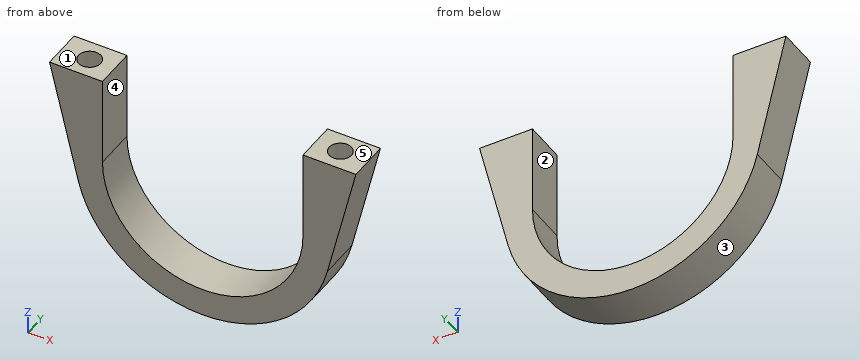
```python
from build123d import *

# Parameters (mm, degrees)
BOSS_EXTRUDE1_DEPTH = 7.5
SKETCH2_R           = 2
CUT_EXTRUDE1_DEPTH  = 4


with BuildPart() as part:
    # Sketch1 → Boss-Extrude1 (new body)
    with BuildSketch(Plane(origin=(0, 0, 0), x_dir=(1, 0, 0), z_dir=(0, 1, 0))):
        with BuildLine():
            Line((-22.363274725, 5.374378434), (-27.5, -16))
            Line((-27.5, -16), (-18, -16))
            Line((-18, -16), (-18, 0))
            ThreePointArc((-18, 0), (0, 18), (18, 0))
            Line((18, 0), (18, -16))
            Line((18, -16), (27.5, -16))
            Line((27.5, -16), (22.363274725, 5.374378434))
            ThreePointArc((22.363274725, 5.374378434), (0, 23), (-22.363274725, 5.374378434))
        make_face()
    extrude(amount=BOSS_EXTRUDE1_DEPTH)

    # Sketch2 → Cut-Extrude1 (cut)
    with BuildSketch(Plane.XY.offset(16)):
        with Locations((-22.5, 3.75)):
            Circle(SKETCH2_R)
        with Locations((22.5, 3.75)):
            Circle(SKETCH2_R)
    extrude(amount=-CUT_EXTRUDE1_DEPTH, mode=Mode.SUBTRACT)


solid = part.part
```
The listing builds one solid part. Answer for the finished solid, in the listing's coordinates (mm). Face numbers are marked on the shaded views. A direction names the side the tool comes from. Coordinates: 2 decimals unless noted, no trailing zeros. Write each loop counter-clockwise with the first axis right and the second up, starting at its lowest first coordinate (ties: lowest second). Pieces come first, ordered by that corner, then holes. Notation, with made-up numbers: (31.5, 77.25) - (78.5, 77.25) arc R22 cw to (78.5, 105.25) - close; hole circle Ø8 at (55, -22.75). An arc over 180 degrees is marked (long way). Return JSON: item names as keys, results as strings. Group by question number.
Q1. The part is cut by section C-C on x = 0. Write down the section's boundary in (y, z).
Q2. Find the intervals of material crossed by line 1 along Y through (x, z) = (22.5, 14.05); line 2 along X through (y, z) = (7, -2.5); line 3 along X through (y, z) = (3.75, -11), in increasing order. Write a range as [from, to].
Q3. Which of the six approach directions +Z, -Z, +X, -X, +Y, -Y give full straight-line access (tool end or side, diameter ignored) to the marked faces 1 and 2?
Q4. The part is cut by section B-B on z = 8.5. Write down the section's boundary in (x, y), and give its area (3 significant figures).
Q5. Flat-ended cylindrical pins translate along their axes: pin 1 Ø4 at (x, y) = (-20.5, 1.5) entering from -Z; pin 2 Ø1.5 at (x, y) = (-6, 4.5) entering from +Z; pin 3 Ø4 at (y, z) = (2.5, 5.5) entering from -X. Find the tip coordinate at first contact, or state that the pin passes through.
Q6. For a pull along X with two mould halves and no side action, classify the marked faces 3, 4 and 5 as +X half, -X half, draft (parallel to the pull), parting line (faces both ways), or undercut.
Q7. The part is cut by section A-A on y = 3.75. Write down the section's boundary in (x, z).
Q8. The part is cut by section D-D on y = 1. Write down the section's boundary in (x, z).
Evaluation:
{
 "1": {"outline": "(0, -23) - (7.5, -23) - (7.5, -18) - (0, -18) - close"},
 "2": {"line 1": "y = [0, 1.75], [5.75, 7.5]", "line 2": "x = [-23.05, -17.83], [17.83, 23.05]", "line 3": "x = [-20.2, -14.25], [14.25, 20.2]"},
 "3": {"face 1": "+Z, +X, -X, +Y, -Y", "face 2": "+Z, +Y, -Y"},
 "4": {"outline": "(-25.7, 0) - (-18, 0) - (-18, 7.5) - (-25.7, 7.5) - close; (18, 0) - (25.7, 0) - (25.7, 7.5) - (18, 7.5) - close", "area": "115 mm2"},
 "5": {"pin 1": "stops at z = -13.67", "pin 2": "stops at z = -16.69", "pin 3": "stops at x = -25.46"},
 "6": {"face 3": "parting line", "face 4": "undercut", "face 5": "draft"},
 "7": {"outline": "(-27.5, 16) - (-22.36, -5.37) arc R23 ccw to (22.36, -5.37) - (27.5, 16) - (24.5, 16) - (24.5, 12) - (20.5, 12) - (20.5, 16) - (18, 16) - (18, 0) arc R18 cw to (-18, 0) - (-18, 16) - (-20.5, 16) - (-20.5, 12) - (-24.5, 12) - (-24.5, 16) - close"},
 "8": {"outline": "(-27.5, 16) - (-22.36, -5.37) arc R23 ccw to (22.36, -5.37) - (27.5, 16) - (18, 16) - (18, 0) arc R18 cw to (-18, 0) - (-18, 16) - close"}
}
